```python
from build123d import *

# Parameters (mm, degrees)
F1_R     = 1.27
F2_DEPTH = 3.175
F3_DEPTH = 3.175
F5_COUNT = 14
F5_ANGLE = 334.2857142857


# Not quite as in the source:
# - a length typed as a fraction of an inch, garbled in the dataset ("3 / 203.2 mm" for 3/8 in), is restored


with BuildPart() as f2:
    # F1 (on Front) → F2 (new body)
    with BuildSketch(Plane.XZ):
        with BuildLine():
            ThreePointArc((6.6428889328, -0.0990154985), (6.6434423524, -0.049509124), (6.643626829, 0))
            ThreePointArc((6.643626829, 0), (6.5953592641, 0.7993832744), (6.4512579209, 1.587151121))
            ThreePointArc((6.4512579209, 1.587151121), (-6.6011332303, -0.7502116494), (6.6428889328, -0.0990154985))
        make_face()
        Circle(F1_R, mode=Mode.SUBTRACT)
    extrude(amount=F2_DEPTH)

    # F1 (on Front) → F3 (join)
    with BuildSketch(Plane.XZ):
        with BuildLine():
            ThreePointArc((6.4512579209, 1.587151121), (6.5953592641, 0.7993832744), (6.643626829, 0))
            ThreePointArc((6.643626829, 0), (6.6434423524, -0.049509124), (6.6428889328, -0.0990154985))
            ThreePointArc((6.6428889328, -0.0990154985), (7.4027472944, 0.1325210174), (8.0591667411, 0.5798546712))
            ThreePointArc((8.0591667411, 0.5798546712), (8.0283191506, 0.9124097851), (7.9837548494, 1.2434060096))
            ThreePointArc((7.9837548494, 1.2434060096), (7.2436944715, 1.5320312423), (6.4512579209, 1.587151121))
        make_face()
    extrude(amount=F3_DEPTH)

    # F5: F2 ×14 about axis
    f5_axis = Axis((0, 6.1465417966, 0), (0, 1, 0))


with BuildPart() as f2_1:
    add(f2.part)
    for i in range(1, F5_COUNT):
        add(f2.part.rotate(f5_axis, i * F5_ANGLE / (F5_COUNT - 1)))


solid = f2_1.part
```
The model under review builds one solid part; all positions refer to its coordinate system, in mm. A direction names the side the tool comes from. Give positions to 0.01 mm unless a question says otherwise; leave off trailing zeros. Write each loop counter-clockwise with the first axis right and the second up, starting at its lowest first coordinate (ties: lowest second). Pieces come first, ordered by that corner, then holes. Notation, with made-up numbers: M 22,9 L 74,9 A14 ccw 74,34 Z; hole C 31.5,55 d11. An arc over 180 degrees is marked long. Write each question's results on one line, items separated by ' | '. Start each with the question number.
1. For faces 5 (the cylindrical face through (-3.33, -1.57, -6.63)), 6 (the cylindrical face through (5.72, -1.57, -4.72)), 7 (the cylindrical face through (0.12, -1.57, 7.41)), 8 (the cylindrical face through (-7.2, -1.57, 1.77)), list the 3-axis set-ups (+Z, -Z, +X, -X, +Y, -Y) from which the entire face can be reached by the end or side of a thin tool; tool diameter is ignored.
2. We need section C-C (z = -2). Write out the cut boundary in (x, y) (3 decimals), and give its area (3 significant figures).
3. Insertion check: pin 1 Ø1.5 at (x, y) = (6, -0.5) entering from +Z; pin 2 Ø1 at (y, z) = (-1.5, -6) entering from +X. Each pin has a flat end and moves straight along its axis. Give the tip position at first contact, or say it passes through.
4. For probe 1 along X at (y, z) = (-2.9, -5.5); probe 2 along Z at (x, y) = (-1, -0.75); probe 3 along Z at (x, y) = (-5, -0.45), list the stretches that pass through material, from the lowest coordinate up. Write a range as [from, to].
5. Mouldability with a two-part tool opening along Z and no side actions: class faces 1 (the cylindrical face through (4.71, -1.57, -5.7)), 2 (the flat face through (1.5, -3.175, 0.8)), 3 (the cylindrical face through (-5.72, -1.57, 4.72)), 4 (the cylindrical face through (-6.605, -1.565, -3.323)) as released by +Z, released by -Z, zero draft, split by the parting line, or undercut.
6. We need section B-B (z = 3.75). Write out the cut boundary in (x, y) (3 decimals).
7. We need section A-A (x = -5.75). Write out the cut boundary in (y, z) (3 decimals).
Results found:
1) face 5: -Z, +Y, -Y | face 6: +X, +Y, -Y | face 7: +Z, +Y, -Y | face 8: -X, +Y, -Y
2) outline: M -6.335,-3.175 L 7.453,-3.175 L 7.453,0 L -6.335,0 Z | area: 43.8 mm^2
3) pin 1: stops at z = 4.59 | pin 2: stops at x = 5.92
4) probe 1: x = [-4.4, 3.73], [4.37, 5.92] | probe 2: z = [-8.02, -0.78], [0.78, 6.57] | probe 3: z = [-4.37, 5.82]
5) face 1: released by -Z | face 2: zero draft | face 3: undercut | face 4: undercut
6) outline: M -5.484,-3.175 L 6.886,-3.175 L 6.886,0 L -5.484,0 Z
7) outline: M -3.175,-4.495 L 0,-4.495 L 0,3.328 L -3.175,3.328 Z; M -3.175,4.785 L 0,4.785 L 0,5.677 L -3.175,5.677 Z
